from build123d import *

# Parameters (mm, degrees)
SKETCH1_R           = 1.2
SKETCH1_R_2         = 1.6
BOSS_EXTRUDE1_DEPTH = 4
SKETCH2_R           = 1.2
BOSS_EXTRUDE2_DEPTH = 3
SKETCH3_R           = 2.9
BOSS_EXTRUDE3_DEPTH = 2


with BuildPart() as part:
    # Sketch1 → Boss-Extrude1 (new body)
    with BuildSketch(Plane(origin=(0, 0, 0), x_dir=(1, 0, 0), z_dir=(0, 1, 0))):
        with BuildLine():
            Line((24.1, 4), (15.580757363, 4))
            ThreePointArc((15.580757363, 4), (9.184735872, 4.689747372), (3.082823649, 6.727272727))
            ThreePointArc((3.082823649, 6.727272727), (-7.4, 0), (3.082823649, -6.727272727))
            ThreePointArc((3.082823649, -6.727272727), (9.184735872, -4.689747372), (15.580757363, -4))
            Line((15.580757363, -4), (24.1, -4))
            ThreePointArc((24.1, -4), (28.1, 0), (24.1, 4))
        make_face()
        with Locations((19.5, 0)):
            Circle(SKETCH1_R, mode=Mode.SUBTRACT)
        with Locations((23.5, 0)):
            Circle(SKETCH1_R, mode=Mode.SUBTRACT)
        Circle(SKETCH1_R_2, mode=Mode.SUBTRACT)
    extrude(amount=BOSS_EXTRUDE1_DEPTH)

    # Sketch2 → Boss-Extrude2 (add)
    with BuildSketch(Plane(origin=(0, 4, 0), x_dir=(1, 0, 0), z_dir=(0, 1, 0))):
        with BuildLine():
            Line((19.5, 3), (23.5, 3))
            ThreePointArc((23.5, 3), (26.5, 0), (23.5, -3))
            Line((23.5, -3), (19.5, -3))
            ThreePointArc((19.5, -3), (16.5, 0), (19.5, 3))
        make_face()
        with Locations((19.5, 0)):
            Circle(SKETCH2_R, mode=Mode.SUBTRACT)
        with Locations((23.5, 0)):
            Circle(SKETCH2_R, mode=Mode.SUBTRACT)
    extrude(amount=BOSS_EXTRUDE2_DEPTH)

    # Sketch3 → Boss-Extrude3 (add)
    with BuildSketch(Plane(origin=(0, 4, 0), x_dir=(1, 0, 0), z_dir=(0, 1, 0))):
        with BuildLine():
            ThreePointArc((7.4, 0), (6.227876645, 3.996692695), (3.082823649, 6.727272727))
            ThreePointArc((3.082823649, 6.727272727), (-7.4, 0), (3.082823649, -6.727272727))
            ThreePointArc((3.082823649, -6.727272727), (6.227876645, -3.996692695), (7.4, 0))
        make_face()
        Circle(SKETCH3_R, mode=Mode.SUBTRACT)
    extrude(amount=BOSS_EXTRUDE3_DEPTH)


solid = part.part
The listing builds one solid part. Answer for the finished solid, in the listing's coordinates (mm). A direction names the side the tool comes from. Give positions to 0.01 mm unless a question says otherwise; leave off trailing zeros. Write each loop counter-clockwise with the first axis right and the second up, starting at its lowest first coordinate (ties: lowest second). Pieces come first, ordered by that corner, then holes. Notation, with made-up numbers: (86, -14) - (97, -14) arc R31 ccw to (97, 21) - close; hole circle Ø8 at (-22.5, 22.5). An arc over 180 degrees is marked (long way). Use a Markdown table: item, result.
1. Section B-B on x = 0 is taken. Write down the section's boundary in (y, z).
Values follow:
| item | result |
|---|---|
| outline | (0, -7.4) - (6, -7.4) - (6, -2.9) - (4, -2.9) - (4, -1.6) - (0, -1.6) - close; (0, 1.6) - (4, 1.6) - (4, 2.9) - (6, 2.9) - (6, 7.4) - (0, 7.4) - close |
2. Each of these flat-tipped pins is pushed along its axis until it touches: P1, Ø1.5, axis at x = 8.5, z = -0.5, coming from the -Y side; P2, Ø2.5, axis at x = 0, z = 0, coming from the -Y side; P3, Ø2, axis at x = 20.5, y = 1.5, coming from the -Z side; P4, Ø3, axis at x = 17.5, y = 2, coming from the +Z side. Where does it stop, or does it pass through?
Values follow:
| item | result |
|---|---|
| P1 | stops at y = 0 |
| P2 | passes through |
| P3 | stops at z = -4 |
| P4 | stops at z = 4 |
3. For a pull along Z with two mould halves and no side action, classify faces 6 (the flat face through (-0.1, 6, 3.2)), 7 (the flat face through (20, 2, -4)), 8 (the cylindrical face through (-2.9, 5, -0.1)) as released by +Z, released by -Z, zero draft, split by the parting line, or undercut.
Values follow:
| item | result |
|---|---|
| face 6 | zero draft |
| face 7 | released by -Z |
| face 8 | undercut |
4. Section A-A on y = 4.5 is taken. Write down the section's boundary in (x, z), plus the area to 3 significant figures.
Values follow:
| item | result |
|---|---|
| outline | circle Ø14.8 at (0, 0); (19.5, -3) - (23.5, -3) arc R3 ccw to (23.5, 3) - (19.5, 3) arc R3 ccw to start; hole circle Ø5.8 at (0, 0); hole circle Ø2.4 at (19.5, 0); hole circle Ø2.4 at (23.5, 0) |
| area | 189 mm² |
5. Section C-C on z = -0.5 is taken. Write down the section's boundary in (x, y), plus the area to 3 significant figures.
Values follow:
| item | result |
|---|---|
| outline | (-7.38, 0) - (-1.52, 0) - (-1.52, 4) - (-2.86, 4) - (-2.86, 6) - (-7.38, 6) - close; (1.52, 0) - (18.41, 0) - (18.41, 7) - (16.54, 7) - (16.54, 4) - (7.38, 4) - (7.38, 6) - (2.86, 6) - (2.86, 4) - (1.52, 4) - close; (20.59, 0) - (22.41, 0) - (22.41, 7) - (20.59, 7) - close; (24.59, 0) - (28.07, 0) - (28.07, 4) - (26.46, 4) - (26.46, 7) - (24.59, 7) - close |
| area | 147 mm² |
6. A tool of negligible diameter and unlimited length cuts with its end or side. For faces 1 (the cylindrical face through (26.5, 5.5, -0.1)), 2 (the cylindrical face through (16.5, 5.5, 0.1)), 3 (the flat face through (21, 5, -3)), 4 (the flat face through (20, 2, 4)), 5 (the flat face through (22, 5, 3)), from which of +Z, -Z, +X, -X, +Y, -Y can it reach the whole face along a straight path? Write none if from no direction.
Values follow:
| item | result |
|---|---|
| face 1 | +X, +Y |
| face 2 | +Y |
| face 3 | -Z, +X, +Y |
| face 4 | +Z, +X, +Y, -Y |
| face 5 | +Z, +X, +Y |
7. Section D-D on z = 2.5 is taken. Write down the section's boundary in (x, y), plus the area to 3 significant figures.
Values follow:
| item | result |
|---|---|
| outline | (-6.96, 0) - (27.22, 0) - (27.22, 4) - (25.16, 4) - (25.16, 7) - (17.84, 7) - (17.84, 4) - (6.96, 4) - (6.96, 6) - (1.47, 6) - (1.47, 4) - (-1.47, 4) - (-1.47, 6) - (-6.96, 6) - close |
| area | 181 mm² |
8. Find the intervals of material crossed by probe 1 along Z at (x, y) = (0, 1.45); probe 2 along X at (y, z) = (1.5, 0); probe 3 along Z at (x, y) = (0, 5.2), in increasing order. Write a range as from..to.
Values follow:
| item | result |
|---|---|
| probe 1 | z = -7.4..-1.6, 1.6..7.4 |
| probe 2 | x = -7.4..-1.6, 1.6..18.3, 20.7..22.3, 24.7..28.1 |
| probe 3 | z = -7.4..-2.9, 2.9..7.4 |
